from build123d import *

# Parameters (mm, degrees)
BOSS_EXTRUDE1_DEPTH     = 127
SKETCH3_R               = 10.16
CUT_EXTRUDE1_DEPTH      = 127
CHAMFER1_SIZE           = 5.08
SKETCH4_W               = 19.05
SKETCH4_H               = 76.2
CUT_EXTRUDE3_DEPTH      = 1
CUT_EXTRUDE3_DEPTH_BACK = 12.7
FILLET1_R               = 12.7
CUT_EXTRUDE4_DEPTH      = 31.75
FILLET2_R               = 12.7
FILLET3_R               = 12.7
FILLET4_R               = 12.7
FILLET5_R               = 12.7


with BuildPart() as part:
    # Sketch1 → Boss-Extrude1 (new body)
    with BuildSketch(Plane.XY):
        Polygon((0, 0), (0, 50.8), (38.1, 50.8), (76.2, 19.05), (76.2, 0), align=None)
    extrude(amount=BOSS_EXTRUDE1_DEPTH)

    # Sketch3 → Cut-Extrude1 (cut)
    with BuildSketch(Plane(origin=(0, 50.8, 0), x_dir=(1, 0, 0), z_dir=(0, 1, 0))):
        with Locations((19.05, -25.4)):
            Circle(SKETCH3_R)
    extrude(amount=-CUT_EXTRUDE1_DEPTH, mode=Mode.SUBTRACT)

    # Chamfer1
    chamfer1_edges = [part.edges().sort_by_distance(p)[0] for p in [
        (8.89, 50.8, 25.4),
    ]]
    chamfer(chamfer1_edges, length=CHAMFER1_SIZE)

    # Sketch4 → Cut-Extrude3 (cut, two sides)
    with BuildSketch(Plane(origin=(0, 50.8, 0), x_dir=(1, 0, 0), z_dir=(0, 1, 0))) as cut_extrude3_sk:
        with Locations((9.525, -88.9)):
            Rectangle(SKETCH4_W, SKETCH4_H)
    extrude(amount=CUT_EXTRUDE3_DEPTH, mode=Mode.SUBTRACT)
    extrude(cut_extrude3_sk.sketch, amount=-CUT_EXTRUDE3_DEPTH_BACK, mode=Mode.SUBTRACT)

    # Fillet1
    fillet1_edges = [part.edges().sort_by_distance(p)[0] for p in [
        (19.05, 44.45, 50.8),
    ]]
    fillet(fillet1_edges, radius=FILLET1_R)

    # Sketch5 → Cut-Extrude4 (cut)
    with BuildSketch(Plane(origin=(0, 50.8, 0), x_dir=(1, 0, 0), z_dir=(0, 1, 0))):
        with BuildLine():
            Line((76.2, -50.8), (60.198, -50.8))
            ThreePointArc((60.198, -50.8), (47.498, -63.5), (60.198, -76.2))
            Line((60.198, -76.2), (76.2, -76.2))
            Line((76.2, -76.2), (76.2, -50.8))
        make_face()
    extrude(amount=-CUT_EXTRUDE4_DEPTH, mode=Mode.SUBTRACT)

    # Fillet2
    fillet2_edges = [part.edges().sort_by_distance(p)[0] for p in [
        (0, 19.05, 127),
    ]]
    fillet(fillet2_edges, radius=FILLET2_R)

    # Fillet3
    fillet3_edges = [part.edges().sort_by_distance(p)[0] for p in [
        (76.2, 9.525, 127),
    ]]
    fillet(fillet3_edges, radius=FILLET3_R)

    # Fillet4
    fillet4_edges = [part.edges().sort_by_distance(p)[0] for p in [
        (76.2, 9.525, 0),
    ]]
    fillet(fillet4_edges, radius=FILLET4_R)

    # Fillet5
    fillet5_edges = [part.edges().sort_by_distance(p)[0] for p in [
        (0, 25.4, 0),
    ]]
    fillet(fillet5_edges, radius=FILLET5_R)


solid = part.part
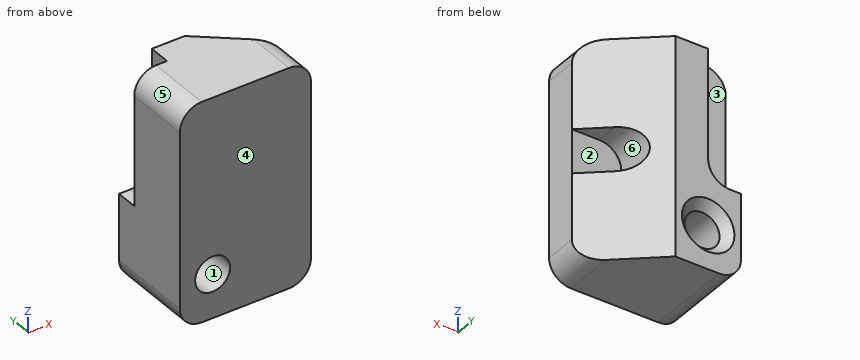
Source: CAD feature listing. Evaluate the final solid. Frame: model axes, mm. Face numbers are marked on the shaded views. A direction names the side the tool comes from. Coordinates: 2 decimals unless noted, no trailing zeros. Write each loop counter-clockwise with the first axis right and the second up, starting at its lowest first coordinate (ties: lowest second). Pieces come first, ordered by that corner, then holes. Notation, with made-up numbers: M 15,67 L 52,67 A9 cw 52,71 Z; hole C -36.5,49.5 d6. An arc over 180 degrees is marked long. Use a Markdown table: item, result.
1) Ray query, L1, parallel to Z at x = 19, y = 10; L2, parallel to X at y = 17.5, z = 25.4; L3, parallel to X at y = 25.5, z = 25.4. Return the intervals inside material, ascending.
Conclusion:
| item | result |
|---|---|
| L1 | z = 0 to 15.24, 35.56 to 127 |
| L2 | x = 0 to 8.89, 29.21 to 76.2 |
| L3 | x = 0 to 8.89, 29.21 to 68.46 |
2) Reachability of the marked faces 1, 2 and 3 from +Z, -Z, +X, -X, +Y, -Y: full face, straight path, thin tool, end or side. Return the list, or none.
Conclusion:
| item | result |
|---|---|
| face 1 | +Y, -Y |
| face 2 | +X, +Y |
| face 3 | +Z, -X, +Y |
3) Section D-D, the plane z = 61.5. Output: boundary loops of the cut face in (x, y).
Conclusion:
| item | result |
|---|---|
| outline | M 0,0 L 76.2,0 L 76.2,19.05 L 47.66,19.05 L 47.66,42.84 L 38.1,50.8 L 18.89,50.8 L 18.89,38.1 L 0,38.1 Z |
4) Mould query, pull axis Z, two halves, no side actions, for the marked faces 4, 5 and 6. Classes: pulls with the +Z half, pulls with the -Z half, needs draft (parallel to the pull), parting line crosses it, or undercut.
Conclusion:
| item | result |
|---|---|
| face 4 | needs draft |
| face 5 | pulls with the +Z half |
| face 6 | undercut |
5) Section A-A, the plane z = 25.4. Output: boundary loops of the cut face in (x, y), then the cut area to 3 significant figures.
Conclusion:
| item | result |
|---|---|
| outline | M 0,0 L 8.89,0 L 8.89,45.72 L 3.81,50.8 L 0,50.8 Z; M 29.21,0 L 76.2,0 L 76.2,19.05 L 38.1,50.8 L 34.29,50.8 L 29.21,45.72 Z |
| area | 2,210 mm^2 |
6) Section B-B, the plane y = 15. Output: boundary loops of the cut face in (x, z).
Conclusion:
| item | result |
|---|---|
| outline | M 0,12.7 A12.7 ccw 12.7,0 L 63.5,0 A12.7 ccw 76.2,12.7 L 76.2,114.3 A12.7 ccw 63.5,127 L 12.7,127 A12.7 ccw 0,114.3 Z; hole C 19.05,25.4 d20.32 |
7) Section C-C, the plane x = 57. Output: boundary loops of the cut face in (y, z), then the cut area to 3 significant figures.
Conclusion:
| item | result |
|---|---|
| outline | M 0,0 L 35.05,0 L 35.05,51.21 L 19.05,51.21 L 19.05,75.79 L 35.05,75.79 L 35.05,127 L 0,127 Z |
| area | 4,060 mm^2 |
8) First-contact query: pin 1 Ø21 at (x, z) = (10.5, 102) entering from +Y; pin 2 Ø6.5 at (x, y) = (70, 24) entering from -Z; pin 3 Ø3 at (x, y) = (10, 12.5) entering from +Z; pin 4 Ø10 at (y, z) = (45.5, 95) entering from -X. Flat tips, straight axial feed; report the tip coordinate or a pass-through.
Conclusion:
| item | result |
|---|---|
| pin 1 | stops at y = 50.8 |
| pin 2 | stops at z = 0.42 |
| pin 3 | stops at z = 126.94 |
| pin 4 | stops at x = 19.05 |
